```python
from build123d import *

# Parameters (mm, degrees)
BOSS_EXTRUDE1_DEPTH                     = 15
F_4_0_4_DIAMETER_HOLE1_D                = 4
CBORE_FOR_M6_HEX_HEAD_BOLT1_D           = 7
CBORE_FOR_M6_HEX_HEAD_BOLT1_CBORE_D     = 25.6
CBORE_FOR_M6_HEX_HEAD_BOLT1_CBORE_DEPTH = 3
SHELL1_DEPTH                            = 5
CUT_EXTRUDE4_START                      = 5
CUT_EXTRUDE4_DEPTH                      = 5
CUT_EXTRUDE5_DEPTH                      = 3
CUT_EXTRUDE5_DEPTH_BACK                 = 3
SKETCH23_R                              = 5
CUT_EXTRUDE6_DEPTH                      = 67.110950493
CUT_EXTRUDE6_DEPTH_BACK                 = 3
FILLET1_R                               = 2
SKETCH30_W                              = 87.8922038
SKETCH30_H                              = 63.386693804
CUT_EXTRUDE8_DEPTH                      = 0.125
SKETCH31_W                              = 82.344977649
SKETCH31_H                              = 39.024548637
CUT_EXTRUDE9_DEPTH                      = 0.125
SKETCH38_R                              = 1.905
CUT_EXTRUDE10_DEPTH                     = 68.319909946
SKETCH39_R                              = 15.3
CUT_EXTRUDE11_DEPTH                     = 7.875


# Read off the part's stored shape, not the designer's step: Shell1
with BuildPart() as part:
    # Sketch1 → Boss-Extrude1 (new body)
    with BuildSketch(Plane(origin=(0, 0, 0), x_dir=(-1, 0, 0), z_dir=(0, 0, -1))):
        with BuildLine():
            Line((-54.628463331, -5.212133486), (-0.593380164, -2.525889334))
            ThreePointArc((-0.593380164, -2.525889334), (12.32206912, 15.671805741), (-8.399323253, 23.953643362))
            Line((-8.399323253, 23.953643362), (-43.781031906, 5.260553383))
            ThreePointArc((-43.781031906, 5.260553383), (-45.231601083, 4.760443022), (-46.765522471, 4.723748524))
            Line((-46.765522471, 4.723748524), (-54.189447973, 5.695292216))
            ThreePointArc((-54.189447973, 5.695292216), (-60.376392814, 0.481764046), (-54.628463331, -5.212133486))
        make_face()
    extrude(amount=-BOSS_EXTRUDE1_DEPTH)

    # Ø4.0 (4) Diameter Hole1 (through all)
    with Locations(Plane(origin=(0, 0, 0), x_dir=(-1, 0, 0), z_dir=(0, 0, -1))):
        with Locations((-54.900567232, 0.261366347)):
            Hole(F_4_0_4_DIAMETER_HOLE1_D / 2)

    # CBORE for M6 Hex Head Bolt1 (through all)
    with Locations(Plane(origin=(0, 0, 0), x_dir=(-1, 0, 0), z_dir=(0, 0, -1))):
        with Locations((-1.298433566, 11.656596333)):
            CounterBoreHole(CBORE_FOR_M6_HEX_HEAD_BOLT1_D / 2, CBORE_FOR_M6_HEX_HEAD_BOLT1_CBORE_D / 2, CBORE_FOR_M6_HEX_HEAD_BOLT1_CBORE_DEPTH)

    # Shell1 outline → Shell1 (cut)
    with BuildSketch(Plane.XY):
        with BuildLine():
            Line((51.170699652, 2.778922273), (47.089922847, 2.244884995))
            ThreePointArc((47.089922847, 2.244884995), (44.789040765, 2.299926742), (42.613186999, 3.050092283))
            Line((42.613186999, 3.050092283), (15.48696558, 17.381590594))
            ThreePointArc((15.48696558, 17.381590594), (16.050757412, 7.599634274), (10.564355185, -0.518488741))
            Line((10.564355185, -0.518488741), (51.385096413, -2.547808785))
            ThreePointArc((51.385096413, -2.547808785), (50.404207808, 0.080391395), (51.170699652, 2.778922273))
        make_face()
    extrude(amount=SHELL1_DEPTH, mode=Mode.SUBTRACT)

    # Sketch21 → Cut-Extrude4 (cut)
    with BuildSketch(Plane(origin=(0, 0, 15), x_dir=(-1, 0, 0), z_dir=(0, 0, -1)).offset(CUT_EXTRUDE4_START)):
        with BuildLine():
            Line((-51.170699652, 2.778922273), (-47.089922847, 2.244884995))
            ThreePointArc((-47.089922847, 2.244884995), (-44.789040765, 2.299926742), (-42.613186999, 3.050092283))
            Line((-42.613186999, 3.050092283), (-15.48696558, 17.381590594))
            ThreePointArc((-15.48696558, 17.381590594), (-16.050757412, 7.599634274), (-10.564355185, -0.518488741))
            Line((-10.564355185, -0.518488741), (-51.385096413, -2.547808785))
            ThreePointArc((-51.385096413, -2.547808785), (-50.404207808, 0.080391395), (-51.170699652, 2.778922273))
        make_face()
    extrude(amount=-CUT_EXTRUDE4_DEPTH, mode=Mode.SUBTRACT)

    # Sketch23 → Cut-Extrude5 (cut, two sides: drawn at the far end of the back side and taken through both)
    with BuildSketch(Plane(origin=(0, 0, 7.5), x_dir=(-1, 0, 0), z_dir=(0, 0, -1)).offset(-CUT_EXTRUDE5_DEPTH_BACK)):
        with Locations((-65.267572651, 7.904637809)):
            Circle(SKETCH23_R)
        Polygon((2.769070011, 26.390627774), (-44.049268023, 5.128933961), (-46.116721719, 9.681475582), (0.701616314, 30.943169395), align=None)
    extrude(amount=CUT_EXTRUDE5_DEPTH + CUT_EXTRUDE5_DEPTH_BACK, mode=Mode.SUBTRACT)

    # Sketch24 → Cut-Extrude6 (cut, two sides: drawn at the far end of the back side and taken through both)
    with BuildSketch(Plane(origin=(0, 0, 7.5), x_dir=(-1, 0, 0), z_dir=(0, 0, -1)).offset(-CUT_EXTRUDE6_DEPTH_BACK)):
        with BuildLine():
            Line((-9.027257312, 24.978582277), (-13.74014268, 20.838163554))
            ThreePointArc((-13.74014268, 20.838163554), (-20.357630392, 23.419198741), (-14.432959892, 27.337255112))
            Line((-14.432959892, 27.337255112), (-9.027257312, 24.978582277))
        make_face()
    extrude(amount=CUT_EXTRUDE6_DEPTH + CUT_EXTRUDE6_DEPTH_BACK, mode=Mode.SUBTRACT)

    # Fillet1
    fillet1_edges = [part.edges().sort_by_distance(p)[0] for p in [
        (10.564355185, -0.518488741, 2.5),
        (51.170699652, 2.778922273, 2.5),
        (51.385096413, -2.547808785, 2.5),
        (15.48696558, 17.381590594, 2.5),
        (51.170699652, 2.778922273, 12.5),
        (51.385096413, -2.547808785, 12.5),
        (10.564355185, -0.518488741, 12.5),
        (15.48696558, 17.381590594, 12.5),
    ]]
    fillet(fillet1_edges, radius=FILLET1_R)

    # Sketch30 → Cut-Extrude8 (cut)
    with BuildSketch(Plane.XY.offset(15)):
        with Locations((24.760370948, 9.451685766)):
            Rectangle(SKETCH30_W, SKETCH30_H)
    extrude(amount=-CUT_EXTRUDE8_DEPTH, mode=Mode.SUBTRACT)

    # Sketch31 → Cut-Extrude9 (cut)
    with BuildSketch(Plane(origin=(0, 0, 0), x_dir=(-1, 0, 0), z_dir=(0, 0, -1))):
        with Locations((-23.438477607, 10.614160855)):
            Rectangle(SKETCH31_W, SKETCH31_H)
    extrude(amount=-CUT_EXTRUDE9_DEPTH, mode=Mode.SUBTRACT)

    # Sketch38 → Cut-Extrude10 (cut, through all)
    with BuildSketch(Plane.XY.offset(14.875)):
        with Locations((-5.615950455, 18.571806714)):
            Circle(SKETCH38_R)
        with Locations((8.213643947, 18.570980353)):
            Circle(SKETCH38_R)
        with Locations((8.212817586, 4.741385951)):
            Circle(SKETCH38_R)
        with Locations((-5.616776816, 4.742212313)):
            Circle(SKETCH38_R)
    extrude(amount=-CUT_EXTRUDE10_DEPTH, mode=Mode.SUBTRACT)

    # Sketch39 → Cut-Extrude11 (cut)
    with BuildSketch(Plane(origin=(0, 0, 0.125), x_dir=(-1, 0, 0), z_dir=(0, 0, -1))):
        with Locations((-1.298433566, 11.656596333)):
            Circle(SKETCH39_R)
    extrude(amount=-CUT_EXTRUDE11_DEPTH, mode=Mode.SUBTRACT)


solid = part.part
```
Could you check a few things on this model? Use its own coordinates, in mm. A direction names the side the tool comes from. Give positions to 0.01 mm unless a question says otherwise; leave off trailing zeros. Order: outer loops, then holes, each group sorted by start corner. A loop starts at its lowest first (then second) coordinate and runs counter-clockwise, first axis right, second up.
Q1. For faces 5 (the flat face through (15, 11, 14.875)), 6 (the flat face through (50.4, 5.2, 7.4)), 7 (the cylindrical face through (14.854, 20.146, 2.343)), 8 (the flat face through (31.447, -1.557, 12.403)), 9 (the cylindrical face through (44.821, 2.294, 2.528)), which set-ups out of +Z, -Z, +X, -X, +Y, -Y let a thin tool reach every point of the face, with its end or its side?
Q2. If I drill on line 1 along Y through (x, z) = (-5.5, 12.5); line 2 along X through (y, z) = (13.5, 11); line 3 along X through (y, z) = (4, 11), over which ranges is the centre line in solid material (lowest first)?
Q3. Suppose I cut it at B-B, the plane z = 11.75. Write out the boundary of the cut face in (x, y) (3 decimals).
Q4. I'm going to push flat-ended pins straight in: P1, Ø9, axis at x = 24, y = 5.5, coming from the +Z side; P2, Ø2, axis at x = 39.5, z = 10, coming from the +Y side; P3, Ø5, axis at x = -5.62, y = 4.74, coming from the -Z side. Where does each tip first touch, or does it pass through?
Q5. Suppose I cut it at C-C, the plane y = 4. Write out the boundary of the cut face in (x, z) (3 decimals).
Q6. Suppose I cut it at A-A, the plane y = 12.5. Write out the boundary of the cut face in (x, z) (1 decimal).
Q7. We'd pull the mould along Y, two halves only. Please class faces 1 (the flat face through (27.989, -3.888, 7.397)), 2 (the cylindrical face through (52.9, 0.3, 7.6)), 3 (the cylindrical face through (16.084, 7.723, 5.757)), 4 (the cylindrical face through (60.37, 0.61, 7.4)): +Y half, -Y half, draft (parallel to the pull), parting line (faces both ways), or undercut.
Solution:
1. face 5: +Z, +X, -X, +Y, -Y
1. face 6: +Z, -Z, +Y
1. face 7: -Z, +X, +Y
1. face 8: +Z
1. face 9: -Z
2. line 1: y = -0.81 to 2.84, 6.64 to 16.67, 20.47 to 24.12
2. line 2: x = -12.78 to -1.68, 4.27 to 16.5, 22.83 to 28.19
2. line 3: x = -10.66 to -7.37, -3.86 to 6.46, 9.97 to 14.54, 40.82 to 58.91
3. outline: (0.593, -2.526) - (54.628, -5.212) arc R5.48 ccw (long way) to (54.189, 5.695) - (46.766, 4.724) arc R5 cw to (43.781, 5.261) - (8.399, 23.954) arc R14.2 ccw (long way) to start; hole circle Ø3.81 at (-5.617, 4.742); hole circle Ø3.81 at (-5.616, 18.572); hole circle Ø7 at (1.298, 11.657); hole circle Ø3.81 at (8.213, 4.741); hole circle Ø3.81 at (8.214, 18.571); hole (13.526, 2.46) arc R2 ccw to (15.025, -0.74) - (48.335, -2.396) arc R2 ccw to (50.424, -0.196) arc R4.5 cw to (50.402, 0.357) arc R2 ccw to (48.143, 2.383) - (47.09, 2.245) arc R7.5 cw to (42.613, 3.05) - (19.431, 15.298) arc R2 ccw to (16.509, 13.313) arc R15.3 cw to start; hole circle Ø4 at (54.901, 0.261)
4. P1: stops at z = 10
4. P2: stops at y = 7.98
4. P3: stops at z = 8
5. outline: (-10.661, 8) - (-7.371, 8) - (-7.371, 14.875) - (-10.661, 14.875) - close; (-3.862, 8) - (6.458, 8) - (6.458, 14.875) - (-3.862, 14.875) - close; (9.968, 8) - (14.545, 8) - (14.545, 5) - (40.815, 5) - (40.815, 0.125) - (58.908, 0.125) - (58.908, 14.875) - (40.815, 14.875) - (40.815, 10) - (14.545, 10) - (14.545, 14.875) - (9.968, 14.875) - close
6. outline: (-12.9, 8) - (-2.1, 8) - (-2.1, 14.9) - (-12.9, 14.9) - close; (4.7, 8) - (16.6, 8) - (16.6, 5) - (24.7, 5) - (24.7, 0.1) - (30.1, 0.1) - (30.1, 4.5) - (27.8, 4.5) - (27.8, 10.5) - (30.1, 10.5) - (30.1, 14.9) - (24.7, 14.9) - (24.7, 10) - (16.6, 10) - (16.6, 14.9) - (4.7, 14.9) - close
7. face 1: -Y half
7. face 2: undercut
7. face 3: undercut
7. face 4: parting line
